```python
from build123d import *

# Parameters (mm, degrees)
BOSS_EXTRUDE1_DEPTH = 5.08
SKETCH5_R           = 9.6901
CUT_EXTRUDE2_DEPTH  = 2.54
SKETCH6_R           = 6.35
SKETCH6_R_2         = 3.2385
BOSS_EXTRUDE4_DEPTH = 12.7
FILLET1_R           = 2.54
SKETCH8_R           = 1.143
CUT_EXTRUDE3_DEPTH  = 7.62
SKETCH9_R           = 1.905
CUT_EXTRUDE4_DEPTH  = 16.2400001


with BuildPart() as part:
    # Sketch1 → Boss-Extrude1 (new body)
    with BuildSketch(Plane.XY):
        with BuildLine():
            Line((-23.828545778, 14.351), (-16.970545778, 14.351))
            ThreePointArc((-16.970545778, 14.351), (0, 22.225), (16.970545778, 14.351))
            Line((16.970545778, 14.351), (23.828545778, 14.351))
            ThreePointArc((23.828545778, 14.351), (24.367361145, 14.127815367), (24.590545778, 13.589))
            Line((24.590545778, 13.589), (24.590545778, 11.811))
            ThreePointArc((24.590545778, 11.811), (24.367361145, 11.272184633), (23.828545778, 11.049))
            Line((23.828545778, 11.049), (19.283936942, 11.049))
            ThreePointArc((19.283936942, 11.049), (22.225, 0), (19.283936942, -11.049))
            Line((19.283936942, -11.049), (23.828545778, -11.049))
            ThreePointArc((23.828545778, -11.049), (24.367361145, -11.272184633), (24.590545778, -11.811))
            Line((24.590545778, -11.811), (24.590545778, -13.589))
            ThreePointArc((24.590545778, -13.589), (24.367361145, -14.127815367), (23.828545778, -14.351))
            Line((23.828545778, -14.351), (16.970545778, -14.351))
            ThreePointArc((16.970545778, -14.351), (0, -22.225), (-16.970545778, -14.351))
            Line((-16.970545778, -14.351), (-23.828545778, -14.351))
            ThreePointArc((-23.828545778, -14.351), (-24.367361145, -14.127815367), (-24.590545778, -13.589))
            Line((-24.590545778, -13.589), (-24.590545778, -11.811))
            ThreePointArc((-24.590545778, -11.811), (-24.367361145, -11.272184633), (-23.828545778, -11.049))
            Line((-23.828545778, -11.049), (-19.283936942, -11.049))
            ThreePointArc((-19.283936942, -11.049), (-22.225, 0), (-19.283936942, 11.049))
            Line((-19.283936942, 11.049), (-23.828545778, 11.049))
            ThreePointArc((-23.828545778, 11.049), (-24.367361145, 11.272184633), (-24.590545778, 11.811))
            Line((-24.590545778, 11.811), (-24.590545778, 13.589))
            ThreePointArc((-24.590545778, 13.589), (-24.367361145, 14.127815367), (-23.828545778, 14.351))
        make_face()
    extrude(amount=BOSS_EXTRUDE1_DEPTH)

    # Sketch5 → Cut-Extrude2 (cut)
    with BuildSketch(Plane(origin=(0, 0, 0), x_dir=(-1, 0, 0), z_dir=(0, 0, -1))):
        Circle(SKETCH5_R)
    extrude(amount=-CUT_EXTRUDE2_DEPTH, mode=Mode.SUBTRACT)

    # Sketch6 → Boss-Extrude4 (add)
    with BuildSketch(Plane.XY.offset(5.08)):
        Circle(SKETCH6_R)
        Circle(SKETCH6_R_2, mode=Mode.SUBTRACT)
    extrude(amount=BOSS_EXTRUDE4_DEPTH)

    # Fillet1
    fillet1_edges = [part.edges().sort_by_distance(p)[0] for p in [
        (-6.35, 0, 5.08),
    ]]
    fillet(fillet1_edges, radius=FILLET1_R)

    # Sketch8 → Cut-Extrude3 (cut)
    with BuildSketch(Plane(origin=(0, 6.35, 0), x_dir=(1, 0, 0), z_dir=(0, 1, 0))):
        with Locations((0, -12.7)):
            Circle(SKETCH8_R)
    extrude(amount=-CUT_EXTRUDE3_DEPTH, mode=Mode.SUBTRACT)

    # Sketch9 → Cut-Extrude4 (cut, through all)
    with BuildSketch(Plane(origin=(0, 0, 2.54), x_dir=(-1, 0, 0), z_dir=(0, 0, -1))):
        Circle(SKETCH9_R)
    extrude(amount=-CUT_EXTRUDE4_DEPTH, mode=Mode.SUBTRACT)


solid = part.part
```
Verification items for the finished model (mm, model axes). A direction names the side the tool comes from. Coordinates: 2 decimals unless noted, no trailing zeros. Write each loop counter-clockwise with the first axis right and the second up, starting at its lowest first coordinate (ties: lowest second). Pieces come first, ordered by that corner, then holes. Notation, with made-up numbers: M 36,86 L 93,86 A20 cw 93,122 Z; hole C 36,-14 d1. An arc over 180 degrees is marked long. Answer as a JSON object with one key per item and string values. Group by question number.
(1) Release check for a two-part mould opening along Z. For faces 1 (the face through (-0.842, 4.713, 11.928)), 2 (the face through (7.69, -5.896, 1.252)), 3 (the face through (0.1, 2.3, 2.54)) record: +Z half, -Z half, draft (parallel to the pull), parting line (faces both ways), or undercut.
(2) Material ranges on line 1 (Z direction, x = -20, y = 5.5); line 2 (Y direction, x = 0.5, z = 16.5); line 3 (Y direction, x = 1.5, z = 11.5), recorded low to high.
(3) Cross-section at B-B, the plane x = 0. State how many separate pieces and enclosed holes the cut face has, and give its area (3 significant figures).
(4) Cross-section at C-C, the plane z = 14.75. Record the cut outline in (x, y).
(5) Gauge pin test, flat ends, axial feed: pin 1 (3.5 mm diameter, centred on x = 0, y = 0, fed in from -Z); pin 2 (1 mm diameter, centred on y = 5.5, z = 12, fed in from -X); pin 3 (10 mm diameter, centred on x = 17.5, y = -5, fed in from +Z); pin 4 (4 mm diameter, centred on x = -20, z = 3.5, fed in from -Y). Record the tip position at first contact, or that the pin passes through.
(6) Cross-section at D-D, the plane x = 18. Record the cut outline in (y, z).
(7) Tool access check on faces 4 (the face through (-20, 14.351, 3)), 5 (the face through (-22, 11.049, 3)), 6 (the face through (-0.7, -3.16, 11.34)). Record the directions out of +Z, -Z, +X, -X, +Y, -Y that give a thin tool (end or side, any length) a straight path to the whole face; none if there is none.
Reply:
{
 "1": {"face 1": "undercut", "face 2": "draft", "face 3": "-Z half"},
 "2": {"line 1": "0 to 5.08", "line 2": "-6.33 to -3.2, 3.2 to 6.33", "line 3": "-6.17 to -2.87, 2.87 to 6.17"},
 "3": {"separate pieces": "3", "enclosed holes": "0", "area": "242 mm²"},
 "4": {"outline": "C 0,0 d12.7; hole C 0,0 d6.48"},
 "5": {"pin 1": "through", "pin 2": "x = -3.91", "pin 3": "z = 5.08", "pin 4": "y = -14.35"},
 "6": {"outline": "M -14.35,0 L 14.35,0 L 14.35,5.08 L -14.35,5.08 Z"},
 "7": {"face 4": "+Z, -Z, -X, +Y", "face 5": "+Z, -Z, -X", "face 6": "+Z"}
}
